Autodesk Inventor part; units mm, degrees
ref_plane "YZ Plane" through (0, 0, 0) normal (1, 0, 0) x (0, 1, 0)
ref_plane "XZ Plane" through (0, 0, 0) normal (0, 1, 0) x (-1, 0, 0)
ref_plane "XY Plane" through (0, 0, 0) normal (0, 0, 1) x (1, 0, 0)
sketch "スケッチ1" plane through (0, 0, 0) normal (0, 0, 1) x (1, 0, 0)
  point P0 (0, 0)
sketch "スケッチ2" plane through (0, 0, 0) normal (0, 0, 1) x (1, 0, 0)
  line L0 (0, 0) -> (15, 0)
  line L1 (15, 0) -> (15, 30)
  line L2 (15, 30) -> (0, 30)
  line L3 (0, 30) -> (0, 0)
  dimension "d0" = 15
  dimension "d1" = 30
extrude "押し出し1" add sketch "スケッチ2" along normal blind 770
sketch "スケッチ3" plane through (0, 0, 770) normal (0, 0, 1) x (1, 0, 0)
  line L0 (1, 29) -> (14, 29)
  line L1 (14, 29) -> (14, 1)
  line L2 (14, 1) -> (1, 1)
  line L3 (1, 1) -> (1, 29)
  line L4 (0, 30) -> (0, 0)
  line L5 (15, 30) -> (0, 30)
  dimension "d4" = 13
  dimension "d5" = 28
  dimension "d6" = 1
  dimension "d7" = 1
extrude "押し出し2" cut sketch "スケッチ3" against normal blind 770
sketch "スケッチ4" plane through (0, 30, 770) normal (0, 1, 0) x (1, 0, 0)
  circle A0 centre (7.5, 760) radius 1.6
  line L0 (15, 770) -> (0, 770)
  line L1 (15, 770) -> (15, 0)
  circle A1 centre (7.5, 750) radius 1.6
  dimension "d10" = 3.2
  dimension "d11" = 10
  dimension "d12" = 7.5
  dimension "d13" = 3.2
  dimension "d14" = 7.5
  dimension "d15" = 10
sketch "スケッチ5" plane through (0, 30, 770) normal (0, 1, 0) x (1, 0, 0)
  point P0 (0, 770)
hole "穴1" at (7.5, 30, 20) at (7.5, 30, 10) direction (0, -1, 0) diameter 3.4 depth 30
sketch "スケッチ6" plane through (0, 30, 770) normal (0, 1, 0) x (1, 0, 0)
  circle A0 centre (7.5, 750) radius 1.7
  circle A1 centre (7.5, 750) radius 1.7
  point P0 (0, 770)
  dimension "d23" = 3.4
extrude "押し出し3" add sketch "スケッチ6" against normal blind 1
sketch "スケッチ7" plane through (15, 0, 0) normal (0, -1, 0) x (1, 0, 0)
  circle A0 centre (-7.5, 20) radius 1.7
  circle A1 centre (-7.5, 20) radius 1.7
  point P0 (-15, 0)
  dimension "d26" = 3.4
extrude "押し出し4" add sketch "スケッチ7" against normal blind 1
sketch "スケッチ8" plane through (0, 30, 770) normal (0, 1, 0) x (1, 0, 0)
  circle A0 centre (7.5, 745) radius 1.7
  circle A1 centre (7.5, 760) radius 1.7
  line L0 (15, 770) -> (15, 0)
  point P0 (0, 770)
  dimension "d29" = 3.4
  dimension "d30" = 15
  dimension "d31" = 7.5
hole "穴2" at (7.5, 30, 25) direction (0, -1, 0) diameter 3.4 depth 30
equation "\"BendRadius\" = Thickness"
equation "\"BendReliefWidth\" = Thickness"
equation "\"BendReliefDepth\" = 0.5 * Thickness"
equation "\"CornerReliefSize\" = 4 * Thickness"
equation "\"MinimumRemnant\" = 2 * Thickness"
equation "\"TransitionRadius\" = BendRadius"
equation "\"JacobiRadiusSize\" = BendRadius"
equation "\"GapSize\" = Thickness"
properties part number "オムニ_角柱2_N"
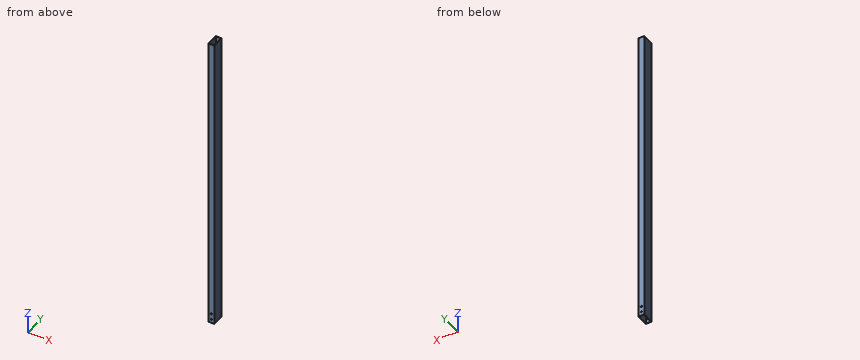
Part model, mm, in its own coordinate system. Coordinates: 2 decimals unless noted, no trailing zeros. Loops run counter-clockwise (first coordinate to the right, second up) from the corner with the lowest first, then second, coordinate; pieces in that order, holes last. Notation, with made-up numbers: (-3, -26.75) - (19, -26.75) arc R13 cw to (19, -13.75) - close; hole circle Ø3 at (-6, -16.75). An arc over 180 degrees is marked (long way). Write item = value, one per line. Start each with the question number.
Item 1: Cut at B-B, the plane y = 14.5. Give the cut face in (x, z), and give its area (3 significant figures).
Item 2: Wall check: L1, parallel to Z at x = 7.5, y = 29.4; L2, parallel to X at y = 0.65, z = 25; L3, parallel to Y at x = 9.25, z = 416. Give the ranges that are in metal, low to high. Write a range as from..to.
Item 3: Cut at A-A, the plane x = 11.75. Give the cut face in (y, z), and give its area (3 significant figures).
Item 4: Cut at C-C, the plane z = 381. Give the cut face in (x, y).
The answers:
q1.outline = (0, 0) - (1, 0) - (1, 770) - (0, 770) - close; (14, 0) - (15, 0) - (15, 770) - (14, 770) - close
q1.area = 1,540 mm2
q2.L1 = 0..8.3, 11.7..23.3, 26.7..770
q2.L2 = 0..5.8, 9.2..15
q2.L3 = 0..1, 29..30
q3.outline = (0, 0) - (1, 0) - (1, 770) - (0, 770) - close; (29, 0) - (30, 0) - (30, 770) - (29, 770) - close
q3.area = 1,540 mm2
q4.outline = (0, 0) - (15, 0) - (15, 30) - (0, 30) - close; hole (1, 1) - (14, 1) - (14, 29) - (1, 29) - close
